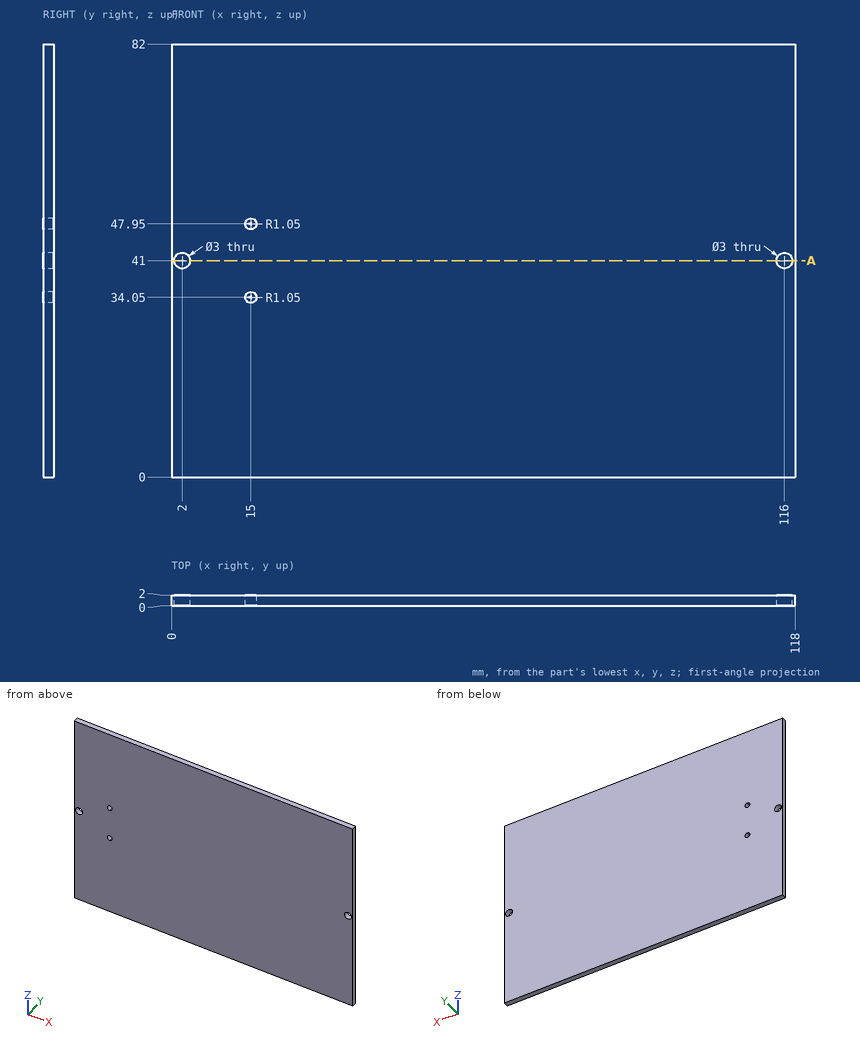
Study the drawing (mm; zero at the part's minimum x, y, z) and answer. Give positions to 0.01 mm unless a question says otherwise; leave off trailing zeros. Loops run counter-clockwise (first coordinate to the right, second up) from the corner with the lowest first, then second, coordinate; pieces in that order, holes last. Notation, with made-up numbers: (36, 56) - (85, 56) arc R9 ccw to (85, 65) - close; hole circle Ø1 at (51.5, 30). An arc over 180 degrees is marked (long way). Return JSON: item names as keys, results as strings. Group by question number.
1. Given pin 1 Ø2.5 at (x, z) = (116, 41) entering from +Y (1 decimal), flat-ended and moving along its own axis, determine where the tip first touches the part or whether it passes through.
2. Find section A-A (z = 41). Write down the section's boundary in (x, y), then the cut area to 3 significant figures.
3. Straight lines are drawn through the part: line 1 (X direction, y = 0.75, z = 41); line 2 (Z direction, x = 2, y = 1); line 3 (X direction, y = 1.8, z = 48). For each, find the intervals that lie inside material, in ascending order. Write a range as [from, to].
Verdict:
{
 "1": {"pin 1": "passes through"},
 "2": {"outline": "(0, 0) - (0.5, 0) - (0.5, 2) - (0, 2) - close; (3.5, 0) - (114.5, 0) - (114.5, 2) - (3.5, 2) - close; (117.5, 0) - (118, 0) - (118, 2) - (117.5, 2) - close", "area": "224 mm^2"},
 "3": {"line 1": "x = [0, 0.5], [3.5, 114.5], [117.5, 118]", "line 2": "z = [0, 39.5], [42.5, 82]", "line 3": "x = [0, 13.95], [16.05, 118]"}
}
